Could you check a few things on this model? Use its own coordinates, in mm. Face numbers are marked on the shaded views. Round coordinates to 2 decimals unless told otherwise and drop trailing zeros. Order: outer loops, then holes, each group sorted by start corner. A loop starts at its lowest first (then second) coordinate and runs counter-clockwise, first axis right, second up. Notation, with made-up numbers: (79.5, -23.75) - (117.5, -23.75) arc R17 cw to (117.5, -4.75) - close; hole circle Ø9 at (1.25, -38). An arc over 180 degrees is marked (long way). Use one line per item in the form item = value.
from build123d import *

# Parameters (mm, degrees)
SKETCH1_R           = 2.65
BOSS_EXTRUDE1_DEPTH = 2
SKETCH4_R           = 15
BOSS_EXTRUDE2_DEPTH = 3
FILLET1_R           = 2
FILLET2_R           = 1


# Read off the part's stored shape, not the designer's step: Shell2
with BuildPart() as part:
    # Sketch1 → Boss-Extrude1 (new body)
    with BuildSketch(Plane(origin=(0, 0, 0), x_dir=(1, 0, 0), z_dir=(0, 1, 0))):
        with BuildLine():
            Line((5, 0), (35, 0))
            ThreePointArc((35, 0), (38.535533906, 1.464466094), (40, 5))
            Line((40, 5), (40, 35))
            ThreePointArc((40, 35), (38.535533906, 38.535533906), (35, 40))
            Line((35, 40), (5, 40))
            ThreePointArc((5, 40), (1.464466094, 38.535533906), (0, 35))
            Line((0, 35), (0, 5))
            ThreePointArc((0, 5), (1.464466094, 1.464466094), (5, 0))
        make_face()
        with Locations(Location((5.5, 34.5, 0), (0, 0, 270))):
            Circle(SKETCH1_R, mode=Mode.SUBTRACT)
        with Locations(Location((34.5, 34.5, 0), (0, 0, 270))):
            Circle(SKETCH1_R, mode=Mode.SUBTRACT)
        with Locations(Location((34.5, 5.5, 0), (0, 0, 270))):
            Circle(SKETCH1_R, mode=Mode.SUBTRACT)
        with Locations(Location((5.5, 5.5, 0), (0, 0, 270))):
            Circle(SKETCH1_R, mode=Mode.SUBTRACT)
    extrude(amount=BOSS_EXTRUDE1_DEPTH)

    # Sketch4 → Boss-Extrude2 (add)
    with BuildSketch(Plane.XZ):
        with Locations(Location((20, -20, 0), (0, 0, 270))):
            Circle(SKETCH4_R)
    extrude(amount=BOSS_EXTRUDE2_DEPTH)

    # Fillet1
    fillet1_edges = [part.edges().sort_by_distance(p)[0] for p in [
        (20, -3, -5),
    ]]
    fillet(fillet1_edges, radius=FILLET1_R)

    # Fillet2
    fillet2_edges = [part.edges().sort_by_distance(p)[0] for p in [
        (20, 0, -5),
    ]]
    fillet(fillet2_edges, radius=FILLET2_R - 0.0001)  # a hair under: the kernel refuses the full size

    # Shell2 outline → Shell2 (revolve, cut)
    with BuildSketch(Plane(origin=(20, 0, -20), x_dir=(1, 0, 0), z_dir=(0, 0, 1))):
        with BuildLine():
            Line((0, -3), (11.968871126, -3))
            ThreePointArc((11.968871126, -3), (11.68272329, -2.269299733), (11.527864045, -1.5))
            Line((11.527864045, -1.5), (0, -1.5))
            Line((0, -1.5), (0, -3))
        make_face()
    revolve(axis=Axis((20, 0, -20), (0, 1, 0)), mode=Mode.SUBTRACT)


solid = part.part
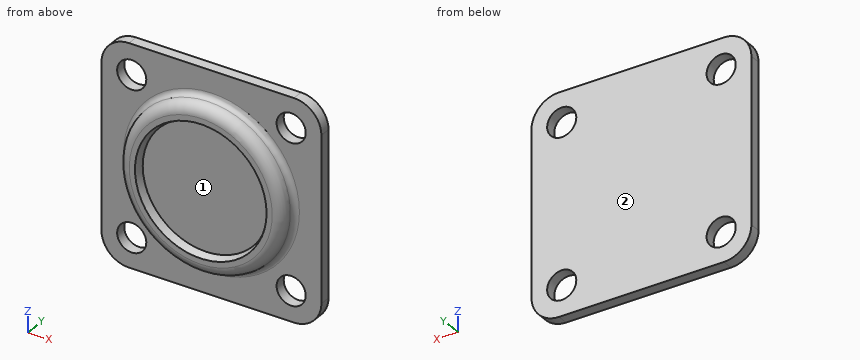
Item 1: Imagine slicing it at A-A on y = 1.1. Please give me the cut outline in (x, z), plus the area to 3 significant figures.
Found:
outline = (0, -35) arc R5 ccw to (5, -40) - (35, -40) arc R5 ccw to (40, -35) - (40, -5) arc R5 ccw to (35, 0) - (5, 0) arc R5 ccw to (0, -5) - close; hole circle Ø5.3 at (5.5, -34.5); hole circle Ø5.3 at (5.5, -5.5); hole circle Ø5.3 at (34.5, -34.5); hole circle Ø5.3 at (34.5, -5.5)
area = 1,490 mm2
Item 2: If we mould it in two halves opening along X, with no side actions, what happens to the marked faces 1 and 2? For each: released by +X, released by -X, zero draft, split by the parting line, or undercut.
Found:
face_1 = undercut
face_2 = zero draft
Item 3: Imagine slicing it at D-D on x = 34.5. State how many separate pieces and enclosed holes the cut face has, plus the area to 3 significant figures.
Found:
separate_pieces = 3
enclosed_holes = 0
area = 76.0 mm2
Item 4: I need wall thicknesses on L1, parallel to X at y = 1.55, z = -5.5; L2, parallel to Y at x = 17.5, z = -13; L3, parallel to X at y = 0.8, z = -36. Which ranges of each line are inside material? Lowest first, please.
Found:
L1 = 0 to 2.85, 8.15 to 31.85, 37.15 to 40
L2 = -1.5 to 2
L3 = 0.1 to 3.32, 7.68 to 32.32, 36.68 to 39.9
Item 5: Will these pins go through, and if not, where does the flat tip stop? P1, Ø8.5, axis at x = 5.5, z = -34.5, coming from the -Y side; P2, Ø3, axis at x = 5.5, z = -5.5, coming from the -Y side; P3, Ø10, axis at x = 4, z = -10.5, coming from the -Y side; P4, Ø7, axis at x = 22, z = -20.5, coming from the -Y side.
Found:
P1 = 0
P2 = through
P3 = -2.91
P4 = -1.5
